Design review of the part built by this model. Coordinates are the model's own, in mm. Round coordinates to 2 decimals unless told otherwise and drop trailing zeros. Order: outer loops, then holes, each group sorted by start corner. A loop starts at its lowest first (then second) coordinate and runs counter-clockwise, first axis right, second up. Notation, with made-up numbers: (17, 56.5) - (43, 56.5) arc R33 ccw to (43, 86.5) - close; hole circle Ø6 at (44.5, 46). An arc over 180 degrees is marked (long way). Write item = value, one per line.
from build123d import *

# Parameters (mm, degrees)
EXTRUDE_1_DEPTH   = 2
HOLE_WIZARD_M51_D = 5.5
CHAMFER_1_SIZE    = 2


with BuildPart() as part:
    # Эскиз1 → Бобышка-Вытянуть1 (new body)
    with BuildSketch(Plane(origin=(0, 0, 0), x_dir=(1, 0, 0), z_dir=(0, 0, -1))):
        Polygon((0, 0), (0, 80), (80, 80), (80, 40), (40, 0), align=None)
    extrude(amount=EXTRUDE_1_DEPTH)

    # Отверстие с зазором M51 (through all)
    with Locations(Plane(origin=(0, 0, -2), x_dir=(1, 0, 0), z_dir=(0, 0, -1))):
        with Locations((10, 70), (10, 50), (10, 30), (10, 10), (30, 70), (30, 50), (30, 30), (30, 10), (50, 70), (50, 50), (70, 70), (70, 50)):
            Hole(HOLE_WIZARD_M51_D / 2)

    # Фаска1
    chamfer_1_edges = [part.edges().sort_by_distance(p)[0] for p in [
        (0, 0, -1),
        (0, -80, -1),
        (80, -80, -1),
    ]]
    chamfer(chamfer_1_edges, length=CHAMFER_1_SIZE)


solid = part.part
1) The part is to be moulded in two halves that separate along X. For faces 1 (the flat face through (60, -20, -1)), 2 (the flat face through (39, -80, -1)), 3 (the cylindrical face through (8.52, -12.32, -0.99)), 4 (the flat face through (1, -79, -1)), say which applies: released by +X, released by -X, zero draft, split by the parting line, or undercut.
Findings:
face_1 = released by +X
face_2 = zero draft
face_3 = undercut
face_4 = released by -X
2) Clearance check with a flat-ended pin moving along its axis: pin 1 Ø1 at (y, z) = (-27.5, -1) entering from +X. State where the tip first meets the part, or that it passes through.
Findings:
pin_1 = 68
3) We need section D-D on x = 50. Write out the cut boundary in (y, z).
Findings:
outline = (-80, -2) - (-72.75, -2) - (-72.75, 0) - (-80, 0) - close; (-67.25, -2) - (-52.75, -2) - (-52.75, 0) - (-67.25, 0) - close; (-47.25, -2) - (-10, -2) - (-10, 0) - (-47.25, 0) - close
4) We need section B-B on z = -0.7. Give the number of separate pieces and of enclosed holes in the cut face, and give its area (3 significant figures).
Findings:
separate_pieces = 1
enclosed_holes = 12
area = 5,310 mm^2
5) We need section A-A on y = -50. Write out the cut boundary in (x, z).
Findings:
outline = (0, -2) - (7.25, -2) - (7.25, 0) - (0, 0) - close; (12.75, -2) - (27.25, -2) - (27.25, 0) - (12.75, 0) - close; (32.75, -2) - (47.25, -2) - (47.25, 0) - (32.75, 0) - close; (52.75, -2) - (67.25, -2) - (67.25, 0) - (52.75, 0) - close; (72.75, -2) - (80, -2) - (80, 0) - (72.75, 0) - close
6) We need section C-C on x = 30. Write out the cut boundary in (y, z).
Findings:
outline = (-80, -2) - (-72.75, -2) - (-72.75, 0) - (-80, 0) - close; (-67.25, -2) - (-52.75, -2) - (-52.75, 0) - (-67.25, 0) - close; (-47.25, -2) - (-32.75, -2) - (-32.75, 0) - (-47.25, 0) - close; (-27.25, -2) - (-12.75, -2) - (-12.75, 0) - (-27.25, 0) - close; (-7.25, -2) - (0, -2) - (0, 0) - (-7.25, 0) - close
7) To check wall thickness, follow L1, parallel to Y at x = 30, z = -1.1; L2, parallel to X at y = -70, z = -0.6; L3, parallel to Y at x = 12, z = -1.45. State the ranges of each line that lie inside material, in increasing order. Write a range as from..to.
Findings:
L1 = -80..-72.75, -67.25..-52.75, -47.25..-32.75, -27.25..-12.75, -7.25..0
L2 = 0..7.25, 12.75..27.25, 32.75..47.25, 52.75..67.25, 72.75..80
L3 = -80..-71.89, -68.11..-51.89, -48.11..-31.89, -28.11..-11.89, -8.11..0
